Input: part model. Units: mm. Frame: model coordinates. Give positions to 0.01 mm unless a question says otherwise; leave off trailing zeros. Order: outer loops, then holes, each group sorted by start corner. A loop starts at its lowest first (then second) coordinate and runs counter-clockwise, first axis right, second up. Notation, with made-up numbers: (7.5, 56) - (45.5, 56) arc R11 ccw to (45.5, 73) - close; hole circle Ø7 at (7, -4). An arc over 180 degrees is marked (long way). Answer in a Markdown table with one row per item. Add a question column.
1. Ray query, line 1 (Y direction, x = 85, z = 3.9); line 2 (X direction, y = -14.75, z = 0.3); line 3 (Y direction, x = 84, z = 0.7). Return the intervals inside material, ascending. Write a range as [from, to].
2. Mould query, pull axis X, two halves, no side actions, for faces 1 (the face through (2.85, -3.01, 2.46)), 2 (the face through (87.586, -16.072, 2.465)), 3 (the face through (166.99, -2.85, 2.46)), 4 (the face through (84, 0, 2)). Classes: released by +X, released by -X, zero draft, split by the parting line, or undercut.
3. Section query A-A on x = 85. Return loops of the section in (y, z).
4. Section query C-C on z = 2.1. Return loops of the section in (x, y).
5. Section query B-B on y = -15. Return loops of the section in (x, z), and give its area (3 significant figures).
```python
from build123d import *

# Parameters (mm, degrees)
ESQUISSE1_R        = 2.8
BOSS_EXTRU_1_DEPTH = 5


with BuildPart() as part:
    # Esquisse1 → Boss.-Extru.1 (new body)
    with BuildSketch(Plane.XY):
        with BuildLine():
            Line((10, 0), (160, 0))
            ThreePointArc((160, 0), (167.071067812, -2.928932188), (170, -10))
            Line((170, -10), (170, -20))
            ThreePointArc((170, -20), (167.071067812, -27.071067812), (160, -30))
            Line((160, -30), (10, -30))
            ThreePointArc((10, -30), (2.928932188, -27.071067812), (0, -20))
            Line((0, -20), (0, -10))
            ThreePointArc((0, -10), (2.928932188, -2.928932188), (10, 0))
        make_face()
        with Locations((85, -15)):
            Circle(ESQUISSE1_R, mode=Mode.SUBTRACT)
    extrude(amount=BOSS_EXTRU_1_DEPTH)


solid = part.part
```
Answer:
| question | item | result |
|---|---|---|
| 1 | line 1 | y = [-30, -17.8], [-12.2, 0] |
| 1 | line 2 | x = [0, 82.21], [87.79, 170] |
| 1 | line 3 | y = [-30, -17.62], [-12.38, 0] |
| 2 | face 1 | released by -X |
| 2 | face 2 | undercut |
| 2 | face 3 | released by +X |
| 2 | face 4 | zero draft |
| 3 | outline | (-30, 0) - (-17.8, 0) - (-17.8, 5) - (-30, 5) - close; (-12.2, 0) - (0, 0) - (0, 5) - (-12.2, 5) - close |
| 4 | outline | (0, -20) arc R10 ccw to (10, -30) - (160, -30) arc R10 ccw to (170, -20) - (170, -10) arc R10 ccw to (160, 0) - (10, 0) arc R10 ccw to (0, -10) - close; hole circle Ø5.6 at (85, -15) |
| 5 | outline | (0, 0) - (82.2, 0) - (82.2, 5) - (0, 5) - close; (87.8, 0) - (170, 0) - (170, 5) - (87.8, 5) - close |
| 5 | area | 822 mm² |
